from build123d import *

# Parameters (mm, degrees)
BOSS_EXTRUDE1_DEPTH = 90
SKETCH2_R           = 65
CUT_EXTRUDE1_DEPTH  = 813.027357612
SKETCH3_R           = 130
CUT_EXTRUDE2_DEPTH  = 813.027357612


with BuildPart() as part:
    # Sketch1 → Boss-Extrude1 (new body)
    with BuildSketch(Plane.XY):
        with BuildLine():
            ThreePointArc((-188.561808316, 233.333333333), (-259.807621135, 150), (-296.353498375, 46.632649519))
            ThreePointArc((-296.353498375, 46.632649519), (-337.006124854, -34.638611198), (-417.120839632, -77.525512861))
            ThreePointArc((-417.120839632, -77.525512861), (-519.615242271, -300), (-275.699483395, -322.474487139))
            ThreePointArc((-275.699483395, -322.474487139), (-198.500979677, -274.536559755), (-107.791690058, -279.965982852))
            ThreePointArc((-107.791690058, -279.965982852), (0, -300), (107.791690058, -279.965982852))
            ThreePointArc((107.791690058, -279.965982852), (198.500979677, -274.536559755), (275.699483395, -322.474487139))
            ThreePointArc((275.699483395, -322.474487139), (519.615242271, -300), (417.120839632, -77.525512861))
            ThreePointArc((417.120839632, -77.525512861), (337.006124854, -34.638611198), (296.353498375, 46.632649519))
            ThreePointArc((296.353498375, 46.632649519), (259.807621135, 150), (188.561808316, 233.333333333))
            ThreePointArc((188.561808316, 233.333333333), (138.505145177, 309.175170954), (141.421356237, 400))
            ThreePointArc((141.421356237, 400), (0, 600), (-141.421356237, 400))
            ThreePointArc((-141.421356237, 400), (-138.505145177, 309.175170954), (-188.561808316, 233.333333333))
        make_face()
    extrude(amount=BOSS_EXTRUDE1_DEPTH)

    # Sketch2 → Cut-Extrude1 (cut, through all)
    with BuildSketch(Plane.XY.offset(90)):
        with Locations((0, 450)):
            Circle(SKETCH2_R)
        with Locations((-389.711431703, -225)):
            Circle(SKETCH2_R)
        with Locations((389.711431703, -225)):
            Circle(SKETCH2_R)
    extrude(amount=-CUT_EXTRUDE1_DEPTH, mode=Mode.SUBTRACT)

    # Sketch3 → Cut-Extrude2 (cut, through all)
    with BuildSketch(Plane.XY.offset(90)):
        Circle(SKETCH3_R)
    extrude(amount=-CUT_EXTRUDE2_DEPTH, mode=Mode.SUBTRACT)


solid = part.part
Build history of the part. All positions in model axes, mm. Coordinates: 2 decimals unless noted, no trailing zeros. Write each loop counter-clockwise with the first axis right and the second up, starting at its lowest first coordinate (ties: lowest second). Pieces come first, ordered by that corner, then holes.
(1) Cut at C-C on y = -225. List the corners of the cut face in (x, z).
(2) Pin check, flat tips, straight feed: pin 1 Ø2 at (y, z) = (340.5, 57) entering from -X; pin 2 Ø1.5 at (y, z) = (472, 45) entering from +X; pin 3 Ø2 at (y, z) = (95.5, 70.5) entering from +X; pin 4 Ø4 at (x, y) = (-218, -4) entering from -Z. Stop position of each tip, or through.
(3) Cut at B-B on x = 0. List the corners of the cut face in (y, z), and give its area (3 significant figures).
(4) Mould opens along Y. For faces 1 (the cylindrical face through (449.755, -249.895, 45.63)), 2 (the cylindrical face through (-259.032, 151.335, 44.37)), 3 (the cylindrical face through (-1.544, -299.996, 44.37)), 4 (the flat face through (-127, 119, 90)) say: pulls with the +Y half, pulls with the -Y half, needs draft (parallel to the pull), parting line crosses it, or undercut.
(5) Cut at D-D on z = 63. List the corners of the cut face in (x, y), and give its area (3 significant figures).
(6) Cut at A-A on y = 450. List the corners of the cut face in (x, z), and give its area (3 significant figures).
(7) Drill centre lines: line 1 (Y direction, x = 0, z = 27.5); line 2 (X direction, y = -211.5, z = 63); line 3 (Y direction, x = -12.5, z = 57.5). Where is each one in solid material? Low to high.
Working result:
1. outline: (-539.71, 0) - (-454.71, 0) - (-454.71, 90) - (-539.71, 90) - close; (-324.71, 0) - (324.71, 0) - (324.71, 90) - (-324.71, 90) - close; (454.71, 0) - (539.71, 0) - (539.71, 90) - (454.71, 90) - close
2. pin 1: stops at x = -133.21
2. pin 2: stops at x = 148.49
2. pin 3: stops at x = 284.73
2. pin 4: stops at z = 0
3. outline: (-300, 0) - (-130, 0) - (-130, 90) - (-300, 90) - close; (130, 0) - (385, 0) - (385, 90) - (130, 90) - close; (515, 0) - (600, 0) - (600, 90) - (515, 90) - close
3. area: 45,900 mm2
4. face 1: undercut
4. face 2: pulls with the +Y half
4. face 3: pulls with the -Y half
4. face 4: needs draft
5. outline: (-417.12, -77.53) arc R150 ccw (long way) to (-275.7, -322.47) arc R150 cw to (-107.79, -279.97) arc R300 ccw to (107.79, -279.97) arc R150 cw to (275.7, -322.47) arc R150 ccw (long way) to (417.12, -77.53) arc R150 cw to (296.35, 46.63) arc R300 ccw to (188.56, 233.33) arc R150 cw to (141.42, 400) arc R150 ccw (long way) to (-141.42, 400) arc R150 cw to (-188.56, 233.33) arc R300 ccw to (-296.35, 46.63) arc R150 cw to start; hole circle Ø130 at (-389.71, -225); hole circle Ø260 at (0, 0); hole circle Ø130 at (0, 450); hole circle Ø130 at (389.71, -225)
5. area: 434,000 mm2
6. outline: (-150, 0) - (-65, 0) - (-65, 90) - (-150, 90) - close; (65, 0) - (150, 0) - (150, 90) - (65, 90) - close
6. area: 15,300 mm2
7. line 1: y = -300 to -130, 130 to 385, 515 to 600
7. line 2: x = -539.1 to -453.29, -326.13 to 326.13, 453.29 to 539.1
7. line 3: y = -299.74 to -129.4, 129.4 to 386.21, 513.79 to 599.48
